Part model, mm, in its own coordinate system. Round coordinates to 2 decimals unless told otherwise and drop trailing zeros. Loops run counter-clockwise (first coordinate to the right, second up) from the corner with the lowest first, then second, coordinate; pieces in that order, holes last.
from build123d import *

# Parameters (mm, degrees)
ESQUISSE1_W             = 62.5
ESQUISSE1_H             = 24.5
BOSS_EXTRU_1_DEPTH      = 4
D_GAGEMENT_M81_D        = 9
ESQUISSE5_R             = 132
ESQUISSE5_R_2           = 57
ENL_V_MAT_EXTRU_1_DEPTH = 73.705605447
D_GAGEMENT_M31_D        = 3.4


with BuildPart() as part:
    # Esquisse1 → Boss.-Extru.1 (new body)
    with BuildSketch(Plane(origin=(0, 0, 0), x_dir=(1, 0, 0), z_dir=(0, 1, 0))):
        Polygon((-58.901607841, -13.53209338), (-58.901607841, 27), (59.427941441, 27), (59.427941441, -12.756380319), (59.427941441, -41.694422162), (-58.901607841, -41.694422162), align=None)
        Rectangle(ESQUISSE1_W, ESQUISSE1_H, mode=Mode.SUBTRACT)
    extrude(amount=BOSS_EXTRU_1_DEPTH)

    # Dégagement M81 (through all)
    with Locations(Plane(origin=(0, 4, 0), x_dir=(1, 0, 0), z_dir=(0, 1, 0))):
        with Locations((-43.3, 19), (43.3, 19)):
            Hole(D_GAGEMENT_M81_D / 2)

    # Esquisse5 → Enlèv. mat.-Extru.1 (cut, through all)
    with BuildSketch(Plane(origin=(0, 4, 0), x_dir=(1, 0, 0), z_dir=(0, 1, 0))):
        with Locations((0, 30)):
            Circle(ESQUISSE5_R)
        with Locations((0, 30)):
            Circle(ESQUISSE5_R_2, mode=Mode.SUBTRACT)
    extrude(amount=-ENL_V_MAT_EXTRU_1_DEPTH, mode=Mode.SUBTRACT)

    # Dégagement M31 (through all)
    with Locations(Plane(origin=(0, 0, 0), x_dir=(-1, 0, 0), z_dir=(0, -1, 0))):
        with Locations((-40, 0), (40, 0)):
            Hole(D_GAGEMENT_M31_D / 2)


solid = part.part
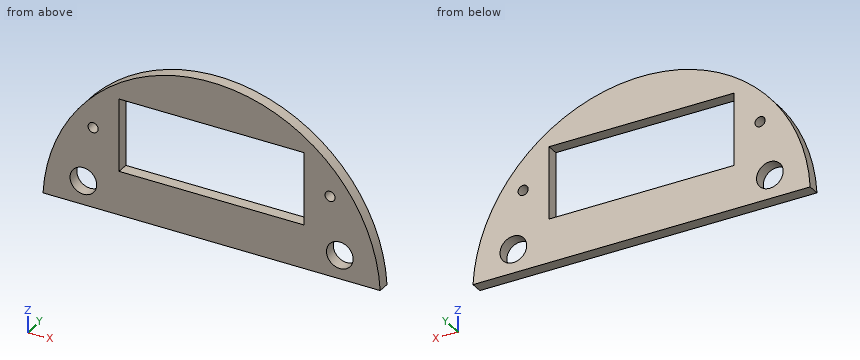
1) Slice it at B-B, the plane x = 14. Give the cut face in (y, z).
Values:
outline: (0, -27) - (4, -27) - (4, -12.25) - (0, -12.25) - close; (0, 12.25) - (4, 12.25) - (4, 25.25) - (0, 25.25) - close
2) Slice it at D-D, the plane z = -21. Give the cut face in (x, y), then the cut area to 3 significant figures.
Values:
outline: (-56.28, 0) - (-47.33, 0) - (-47.33, 4) - (-56.28, 4) - close; (-39.27, 0) - (39.27, 0) - (39.27, 4) - (-39.27, 4) - close; (47.33, 0) - (56.28, 0) - (56.28, 4) - (47.33, 4) - close
area: 386 mm2
3) Wall check: line 1 along Z through (x, y) = (-0.5, 2.5); line 2 along X through (y, z) = (2.1, -19); line 3 along X through (y, z) = (3.2, -7.5). Give the ranges that are in metal, low to high.
Values:
line 1: z = -27 to -12.25, 12.25 to 27
line 2: x = -55.93 to -47.8, -38.8 to 38.8, 47.8 to 55.93
line 3: x = -52.37 to -31.25, 31.25 to 52.37
4) Drop flat-ended pins along their axis: pin 1 Ø1.2 at (x, y) = (-14.5, 3) entering from +Z; pin 2 Ø10 at (x, z) = (-37.5, 13) entering from +Y; pin 3 Ø1.5 at (y, z) = (3, -16) entering from -X; pin 4 Ø2 at (x, z) = (-40, 0) entering from +Y. Give the stop position or say it passes through.
Values:
pin 1: stops at z = 25.28
pin 2: stops at y = 4
pin 3: stops at x = -55.44
pin 4: passes through
5) Slice it at A-A, the plane z = 10. Give the cut face in (x, y).
Values:
outline: (-40.61, 0) - (-31.25, 0) - (-31.25, 4) - (-40.61, 4) - close; (31.25, 0) - (40.61, 0) - (40.61, 4) - (31.25, 4) - close
6) Slice it at C-C, the plane y = 2.8. Give the cut face in (x, z).
Values:
outline: (-56.92, -27) - (56.92, -27) arc R57 ccw to start; hole circle Ø9 at (-43.3, -19); hole circle Ø3.4 at (-40, 0); hole (-31.25, -12.25) - (31.25, -12.25) - (31.25, 12.25) - (-31.25, 12.25) - close; hole circle Ø3.4 at (40, 0); hole circle Ø9 at (43.3, -19)
